Part print with two shaded views. Sizes in mm from the minimum x, y, z corner. A direction names the side the tool comes from. Give positions to 0.01 mm unless a question says otherwise; leave off trailing zeros. Write each loop counter-clockwise with the first axis right and the second up, starting at its lowest first coordinate (ties: lowest second). Pieces come first, ordered by that corner, then holes. Notation, with made-up numbers: (-28.75, 1) -> (5.25, 1) arc R23 ccw to (5.25, 22) -> close; hole circle Ø7 at (45.25, -37.75). An arc over 180 degrees is marked (long way). Answer as a JSON object with one key per item and string values.
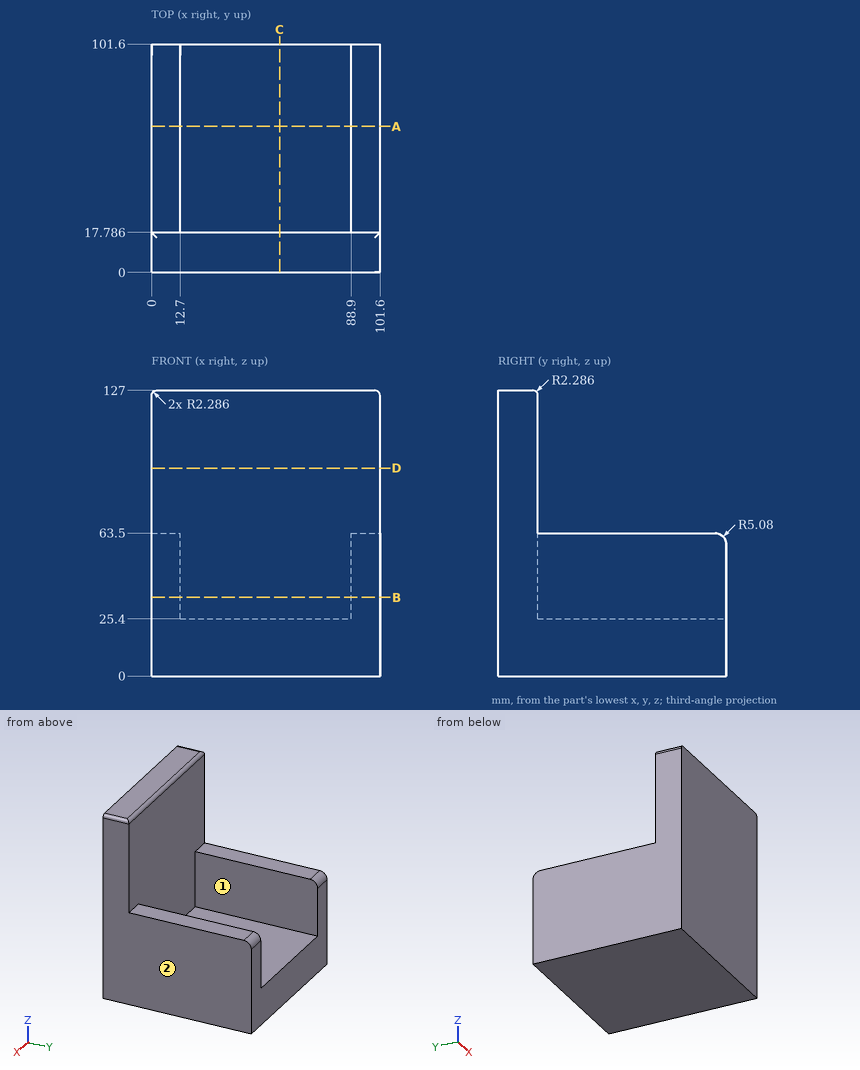
1) Wall check: probe 1 along X at (y, z) = (55, 58); probe 2 along Z at (x, y) = (35.5, 92); probe 3 along Y at (x, z) = (68, 31.5). Give the ranges that are in metal, low to high.
Model answer:
{"probe 1": "x = 0 to 12.7, 88.9 to 101.6", "probe 2": "z = 0 to 25.4", "probe 3": "y = 0 to 17.79"}
2) Pin check, flat tips, straight feed: pin 1 (5 mm diameter, centred on x = 15, z = 90, fed in from +Y); pin 2 (10 mm diameter, centred on x = 6.5, y = 65, fed in from +Z); pin 3 (1.5 mm diameter, centred on x = 13.5, y = 87.5, fed in from +Z). Stop position of each tip, or through.
Model answer:
{"pin 1": "stops at y = 17.79", "pin 2": "stops at z = 63.5", "pin 3": "stops at z = 25.4"}
3) Slice it at D-D (z = 92.5). List the corners of the cut face in (x, y), then the cut area to 3 significant figures.
Model answer:
{"outline": "(0, 0) -> (101.6, 0) -> (101.6, 17.79) -> (0, 17.79) -> close", "area": "1,810 mm2"}
4) Slice it at C-C (x = 57). List the corners of the cut face in (y, z), then the cut area to 3 significant figures.
Model answer:
{"outline": "(0, 0) -> (101.6, 0) -> (101.6, 25.4) -> (17.79, 25.4) -> (17.79, 124.71) arc R2.29 ccw to (15.5, 127) -> (0, 127) -> close", "area": "4,390 mm2"}
5) Slice it at A-A (y = 65). List the corners of the cut face in (x, z).
Model answer:
{"outline": "(0, 0) -> (101.6, 0) -> (101.6, 63.5) -> (88.9, 63.5) -> (88.9, 25.4) -> (12.7, 25.4) -> (12.7, 63.5) -> (0, 63.5) -> close"}
6) Slice it at B-B (z = 35). List the corners of the cut face in (x, y), then the cut area to 3 significant figures.
Model answer:
{"outline": "(0, 0) -> (101.6, 0) -> (101.6, 101.6) -> (88.9, 101.6) -> (88.9, 17.79) -> (12.7, 17.79) -> (12.7, 101.6) -> (0, 101.6) -> close", "area": "3,940 mm2"}
7) 3-axis set-ups, long thin cutter, end or side, ignore diameter. For the marked faces 1 and 2: which of +Z, -Z, +X, -X, +Y, -Y reach the whole face in a straight line?
Model answer:
{"face 1": "+Z, +Y", "face 2": "+Z, -Z, +X, +Y, -Y"}
